Design review of the part built by this model. Coordinates are the model's own, in mm. Face numbers are marked on the shaded views. A direction names the side the tool comes from. Coordinates: 2 decimals unless noted, no trailing zeros. Loops run counter-clockwise (first coordinate to the right, second up) from the corner with the lowest first, then second, coordinate; pieces in that order, holes last. Notation, with made-up numbers: M -28,-4.5 L 21,-4.5 A28 cw 21,17.5 Z; hole C -3.5,54 d3. An arc over 180 degrees is marked long. Put each result on its own line as item: value. Start each with the question number.
(1) Take a section at B-B, the plane x = 3.75. Give the boundary of the cut face in (y, z), then the cut area to 3 significant figures.
(2) Take a section at C-C, the plane y = 2. Give the boundary of the cut face in (x, z).
(3) The part is to be moulded in two halves that separate along Y. For the marked faces 1, 2 and 3, say which applies: +Y half, -Y half, draft (parallel to the pull), parting line (faces both ways), or undercut.
(4) For probe 1 along Y at (x, z) = (-3.75, 1.5); probe 2 along Y at (x, z) = (-6.25, 0.25); probe 3 along Z at (x, y) = (-0.75, 2.75), list the stretches that pass through material, from the lowest coordinate up. Write a range as [from, to].
(5) Take a section at D-D, the plane z = -4. Give the boundary of the cut face in (x, y).
(6) Clearance check with flat-ended pins moving along their axes: pin 1 (1.5 mm diameter, centred on x = 2.5, z = -1, fed in from -Y); pin 2 (6 mm diameter, centred on y = 10.5, z = 3.5, fed in from +X). State where each tip first meets the part, or that it passes through.
(7) For the marked faces 4, 5 and 6, list the 3-axis set-ups (+Z, -Z, +X, -X, +Y, -Y) from which the entire face can be reached by the end or side of a thin tool; tool diameter is ignored.
(8) Take a section at A-A, the plane z = -3. Give the boundary of the cut face in (x, y), then the cut area to 3 significant figures.
```python
from build123d import *

# Parameters (mm, degrees)
SKETCH_1_R          = 5
EXTRUDE_1_DEPTH     = 6
EXTRUDE_START       = 6
SKETCH_1_3_R        = 5
EXTRUDE_2_DEPTH     = 4
EXTRUDE_START_2     = 10
SKETCH_1_4_R        = 5
EXTRUDE_3_DEPTH     = 4
CUT_EXTRUDE_1_DEPTH = 3


with BuildPart() as part:
    # 草图1 → 凸台-拉伸1 (new body)
    with BuildSketch(Plane(origin=(0, 0, 0), x_dir=(1, 0, 0), z_dir=(0, 1, 0))):
        Circle(SKETCH_1_R)
    extrude(amount=EXTRUDE_1_DEPTH)

    # 草图1<3> → 凸台-拉伸2 (add)
    with BuildSketch(Plane(origin=(0, 0, 0), x_dir=(1, 0, 0), z_dir=(0, 1, 0)).offset(EXTRUDE_START)):
        with Locations((-2, 0)):
            Circle(SKETCH_1_3_R)
    extrude(amount=EXTRUDE_2_DEPTH)

    # 草图1<4> → 凸台-拉伸3 (add)
    with BuildSketch(Plane(origin=(0, 0, 0), x_dir=(1, 0, 0), z_dir=(0, 1, 0)).offset(EXTRUDE_START_2)):
        Circle(SKETCH_1_4_R)
    extrude(amount=EXTRUDE_3_DEPTH)

    # 草图2 → 切除-拉伸1 (cut)
    with BuildSketch(Plane.XZ):
        with BuildLine():
            Line((-4.330127019, 2.5), (4.330127019, 2.5))
            ThreePointArc((4.330127019, 2.5), (5, 0), (4.330127019, -2.5))
            Line((4.330127019, -2.5), (-4.330127019, -2.5))
            ThreePointArc((-4.330127019, -2.5), (-5, 0), (-4.330127019, 2.5))
        make_face()
    extrude(amount=-CUT_EXTRUDE_1_DEPTH, mode=Mode.SUBTRACT)


solid = part.part
```
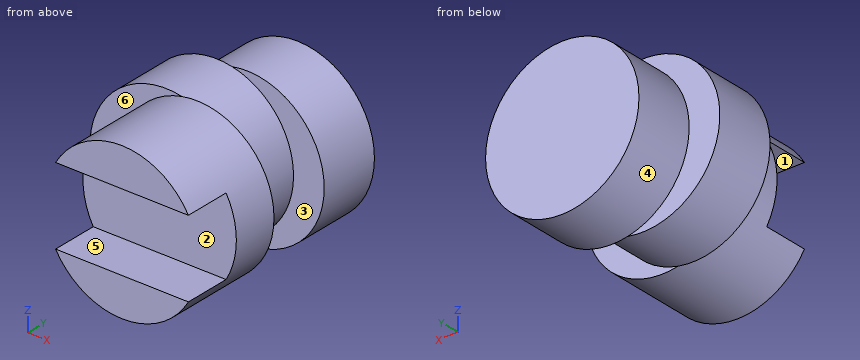
Computed values:
1. outline: M 0,-3.31 L 6,-3.31 L 6,3.31 L 0,3.31 L 0,2.5 L 3,2.5 L 3,-2.5 L 0,-2.5 Z; M 10,-3.31 L 14,-3.31 L 14,3.31 L 10,3.31 Z
1. area: 51.1 mm^2
2. outline: M -4.33,-2.5 A5 ccw 4.33,-2.5 Z; M -4.33,2.5 L 4.33,2.5 A5 ccw Z
3. face 1: draft
3. face 2: -Y half
3. face 3: undercut
4. probe 1: y = [3, 14]
4. probe 2: y = [6, 10]
4. probe 3: z = [-4.94, -2.5], [2.5, 4.94]
5. outline: M -5,6 L -3,6 L -3,0 L 3,0 L 3,6 L 1,6 L 1,10 L 3,10 L 3,14 L -3,14 L -3,10 L -5,10 Z
6. pin 1: stops at y = 3
6. pin 2: stops at x = 4.97
7. face 4: +Y
7. face 5: +X, -X, -Y
7. face 6: -X, -Y
8. outline: M -6,6 L -4,6 L -4,0 L 4,0 L 4,6 L 2,6 L 2,10 L 4,10 L 4,14 L -4,14 L -4,10 L -6,10 Z
8. area: 112 mm^2
